Job drawing, mm, ordinate dimensions from the low corner. One solid piece. A direction names the side the tool comes from. Give positions to 0.01 mm unless a question says otherwise; leave off trailing zeros. Write each loop counter-clockwise with the first axis right and the second up, starting at its lowest first coordinate (ties: lowest second). Pieces come first, ordered by that corner, then holes. Notation, with made-up numbers: (44.5, 55.25) - (83.5, 55.25) arc R9 ccw to (83.5, 66.25) - close; hole circle Ø3 at (-12.5, 41.25). An arc over 180 degrees is marked (long way). Put each result on its own line as item: value. Start each with the question number.
1. Wall check: line 1 (X direction, y = 22.65, z = 18); line 2 (Y direction, x = 15, z = 4.5); line 3 (X direction, y = 22.8, z = 33). Give the ranges that are in metal, low to high.
2. Drop flat-ended pins along their axis: pin 1 (4 mm diameter, centred on x = 18, y = 8.5, fed in from -Z); pin 2 (0.9 mm diameter, centred on x = 17.5, z = 33, fed in from -Y); pin 3 (8 mm diameter, centred on y = 25.5, z = 21, fed in from +X). Give the stop position or say it passes through.
3. Cut at D-D on z = 33. List the corners of the cut face in (x, y).
4. Cut at C-C on y = 13.5. List the corners of the cut face in (x, z), and give its area (3 significant figures).
5. Cut at A-A on z = 18. List the corners of the cut face in (x, y).
6. Tool access for the marked faces 1, 2 and 3: list every direction of +Z, -Z, +X, -X, +Y, -Y with a clear straight run to the whole face (end or side of a thin tool).
7. Cut at B-B on x = 18. List the corners of the cut face in (y, z), and give its area (3 significant figures).
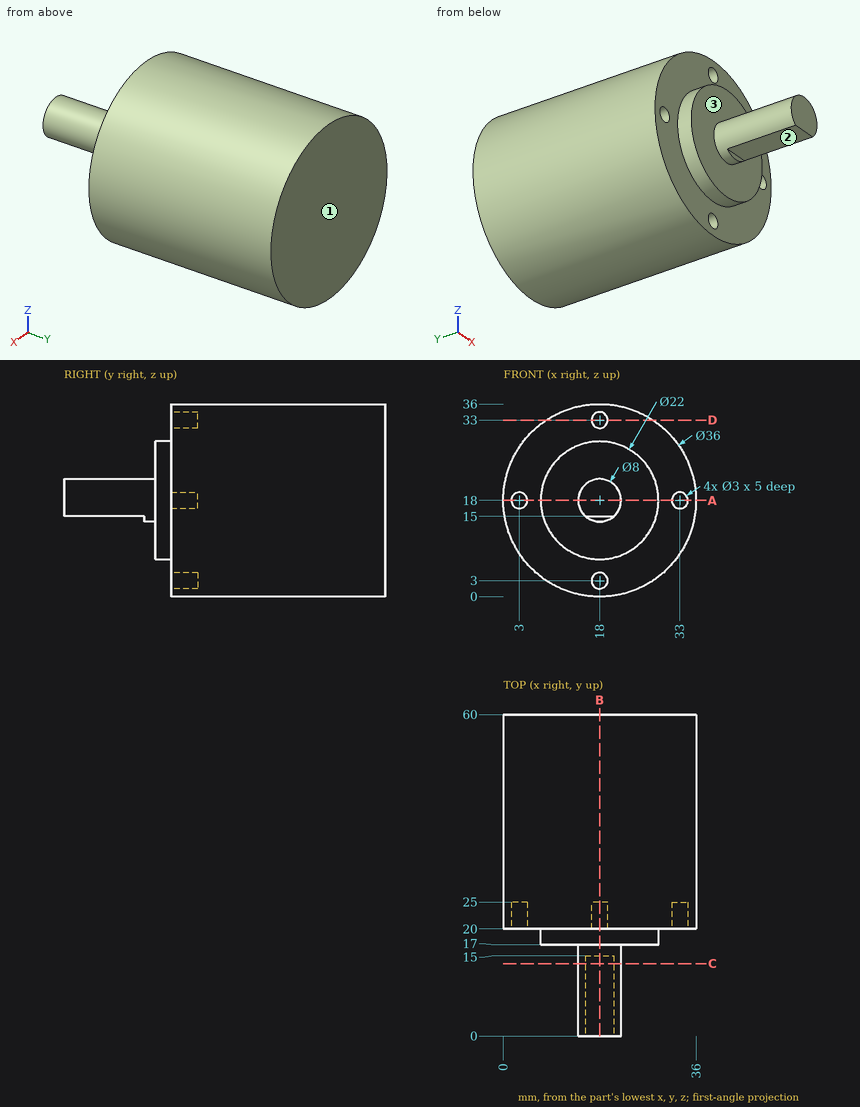
Report:
1. line 1: x = 0 to 1.5, 4.5 to 31.5, 34.5 to 36
1. line 2: y = 20 to 60
1. line 3: x = 8.05 to 16.5, 19.5 to 27.95
2. pin 1: stops at z = 15
2. pin 2: stops at y = 25
2. pin 3: stops at x = 36
3. outline: (8.05, 20) - (16.5, 20) - (16.5, 25) - (19.5, 25) - (19.5, 20) - (27.95, 20) - (27.95, 60) - (8.05, 60) - close
4. outline: (15.35, 15) - (20.65, 15) arc R4 ccw (long way) to start
4. area: 46.6 mm²
5. outline: (0, 20) - (1.5, 20) - (1.5, 25) - (4.5, 25) - (4.5, 20) - (7, 20) - (7, 17) - (14, 17) - (14, 0) - (22, 0) - (22, 17) - (29, 17) - (29, 20) - (31.5, 20) - (31.5, 25) - (34.5, 25) - (34.5, 20) - (36, 20) - (36, 60) - (0, 60) - close
6. face 1: +Z, -Z, +X, -X, +Y
6. face 2: -Z, +X, -X, -Y
6. face 3: -Y
7. outline: (0, 15) - (15, 15) - (15, 14) - (17, 14) - (17, 7) - (20, 7) - (20, 4.5) - (25, 4.5) - (25, 1.5) - (20, 1.5) - (20, 0) - (60, 0) - (60, 36) - (20, 36) - (20, 34.5) - (25, 34.5) - (25, 31.5) - (20, 31.5) - (20, 29) - (17, 29) - (17, 22) - (0, 22) - close
7. area: 1,600 mm²
